Answer from the drawing. Dimensions are ordinates in mm from the lowest x, y and z of the part. Give positions to 0.01 mm unless a question says otherwise; leave off trailing zeros. Write each loop counter-clockwise with the first axis right and the second up, starting at its lowest first coordinate (ties: lowest second). Pieces come first, ordered by that corner, then holes. Notation, with made-up numbers: (56, 64.25) -> (82, 64.25) arc R33 cw to (82, 103.25) -> close; hole circle Ø4 at (84, -24). An arc over 180 degrees is marked (long way). Write item = value, one per line.
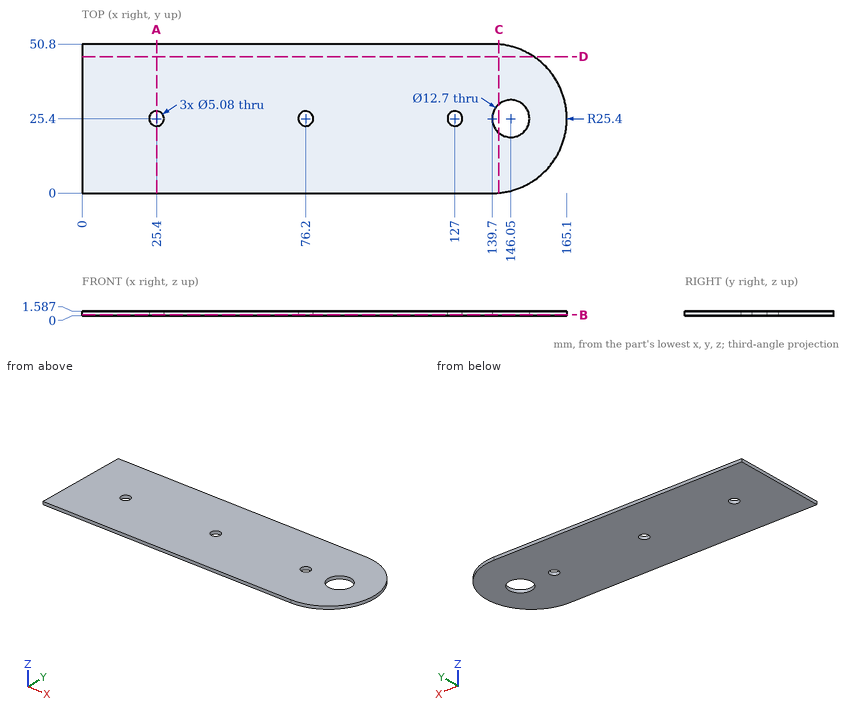
(1) The part is cut by section B-B on z = 0.3. Determine the outline of the cut face in (x, y), plus the area to 3 significant figures.
Checks:
outline = (0, 0) -> (139.7, 0) arc R25.4 ccw to (139.7, 50.8) -> (0, 50.8) -> close; hole circle Ø5.08 at (25.4, 25.4); hole circle Ø5.08 at (76.2, 25.4); hole circle Ø5.08 at (127, 25.4); hole circle Ø12.7 at (146.05, 25.4)
area = 7,920 mm²
(2) The part is cut by section C-C on x = 142. Determine the outline of the cut face in (y, z) (1 decimal).
Checks:
outline = (0.1, 0) -> (20.5, 0) -> (20.5, 1.6) -> (0.1, 1.6) -> close; (30.3, 0) -> (50.7, 0) -> (50.7, 1.6) -> (30.3, 1.6) -> close
(3) The part is cut by section D-D on y = 46.5. Determine the outline of the cut face in (x, z).
Checks:
outline = (0, 0) -> (153.84, 0) -> (153.84, 1.59) -> (0, 1.59) -> close
(4) Consider L1, parallel to Y at x = 76.2, z = 0.4; L2, parallel to Y at x = 74.5, z = 1.45 (1 decimal); L3, parallel to X at y = 31, z = 0.55 (1 decimal). Determine where each line is inside the solid, lowest interval first.
Checks:
L1 = 0 to 22.86, 27.94 to 50.8
L2 = 0 to 23.5, 27.3 to 50.8
L3 = 0 to 143.1, 149 to 164.5
(5) The part is cut by section A-A on x = 25.4. Determine the outline of the cut face in (y, z).
Checks:
outline = (0, 0) -> (22.86, 0) -> (22.86, 1.59) -> (0, 1.59) -> close; (27.94, 0) -> (50.8, 0) -> (50.8, 1.59) -> (27.94, 1.59) -> close
